Geometry check sheet. Reference: the model listing, model coordinates, mm. Face numbers are marked on the shaded views. A direction names the side the tool comes from. Give positions to 0.01 mm unless a question says otherwise; leave off trailing zeros. Loops run counter-clockwise (first coordinate to the right, second up) from the corner with the lowest first, then second, coordinate; pieces in that order, holes last. Notation, with made-up numbers: (76.25, 31.5) -> (81.25, 31.5) arc R20 cw to (81.25, 58.5) -> close; hole circle Ø1 at (-31.5, -27). An arc over 180 degrees is marked (long way). Write item = value, one per line. Start each with the question number.
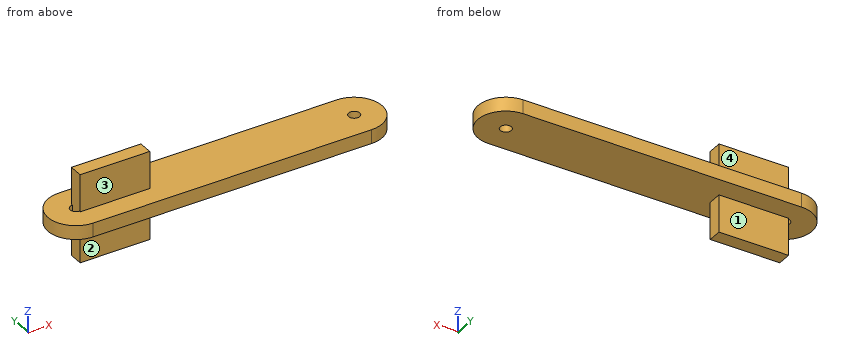
```python
from build123d import *

# Parameters (mm, degrees)
BOSS_EXTRUDE1_DEPTH      = 2.5
BOSS_EXTRUDE1_DEPTH_BACK = 2.5
SKETCH1_R                = 2
BOSS_EXTRUDE2_START      = -50
SKETCH2_W                = 31.75
SKETCH2_H                = 5
BOSS_EXTRUDE2_DEPTH      = 25


with BuildPart() as part:
    # Sketch1 → Boss-Extrude1 (new, two sides: drawn at the far end of the back side and taken through both)
    with BuildSketch(Plane.XY.offset(-BOSS_EXTRUDE1_DEPTH_BACK)):
        with BuildLine():
            Line((-50, 10), (50, 10))
            ThreePointArc((50, 10), (60, 0), (50, -10))
            Line((50, -10), (-50, -10))
            ThreePointArc((-50, -10), (-60, 0), (-50, 10))
        make_face()
        with Locations((-50, 0)):
            Circle(SKETCH1_R, mode=Mode.SUBTRACT)
        with Locations((50, 0)):
            Circle(SKETCH1_R, mode=Mode.SUBTRACT)
    extrude(amount=BOSS_EXTRUDE1_DEPTH + BOSS_EXTRUDE1_DEPTH_BACK)

    # Sketch2 → Boss-Extrude2 (add)
    with BuildSketch(Plane(origin=(0, 0, 0), x_dir=(0, 0, -1), z_dir=(1, 0, 0)).offset(BOSS_EXTRUDE2_START)):
        Rectangle(SKETCH2_W, SKETCH2_H)
    extrude(amount=BOSS_EXTRUDE2_DEPTH)


solid = part.part
```
1) Section check D-D (x = 40). Enter the section's corners in (y, z), plus the area to 3 significant figures.
2) Section check C-C (z = 7). Enter the section's corners in (x, y), plus the area to 3 significant figures.
3) Section check A-A (y = 0). Enter the section's corners in (x, z) (3 decimals).
4) Thickness scan on line 1 (Y direction, x = 50, z = -1); line 2 (Z direction, x = 0, y = -5.75); line 3 (X direction, y = 1, z = -12). Record the ranges inside material, lowest first.
5) Tool access check on the marked faces 1, 2, 3 and 4. Record the directions out of +Z, -Z, +X, -X, +Y, -Y that give a thin tool (end or side, any length) a straight path to the whole face; none if there is none.
6) Section check B-B (x = -32). Enter the section's corners in (y, z) (3 decimals), plus the area to 3 significant figures.
7) Depth check by flat-ended pin: pin 1 Ø1.5 at (y, z) = (1, -7) entering from +X; pin 2 Ø3 at (y, z) = (5.5, -7.5) entering from +X; pin 3 Ø1.5 at (x, z) = (-27.5, -7) entering from +Y; pin 4 Ø1.5 at (y, z) = (-1, 4) entering from -X. Enter the tip coordinate at first touch or a pass-through.
Check result:
q1.outline = (-10, -2.5) -> (10, -2.5) -> (10, 2.5) -> (-10, 2.5) -> close
q1.area = 100 mm2
q2.outline = (-50, -2.5) -> (-25, -2.5) -> (-25, 2.5) -> (-50, 2.5) -> close
q2.area = 125 mm2
q3.outline = (-60, -2.5) -> (-52, -2.5) -> (-52, 2.5) -> (-60, 2.5) -> close; (-50, -15.875) -> (-25, -15.875) -> (-25, -2.5) -> (48, -2.5) -> (48, 2.5) -> (-25, 2.5) -> (-25, 15.875) -> (-50, 15.875) -> close; (52, -2.5) -> (60, -2.5) -> (60, 2.5) -> (52, 2.5) -> close
q4.line_1 = -10 to -2, 2 to 10
q4.line_2 = -2.5 to 2.5
q4.line_3 = -50 to -25
q5.face_1 = -Z, +X, -X, +Y
q5.face_2 = -Z, +X, -X, -Y
q5.face_3 = +Z, +X, -X, -Y
q5.face_4 = +Z, +X, -X, +Y
q6.outline = (-10, -2.5) -> (-2.5, -2.5) -> (-2.5, -15.875) -> (2.5, -15.875) -> (2.5, -2.5) -> (10, -2.5) -> (10, 2.5) -> (2.5, 2.5) -> (2.5, 15.875) -> (-2.5, 15.875) -> (-2.5, 2.5) -> (-10, 2.5) -> close
q6.area = 234 mm2
q7.pin_1 = -25
q7.pin_2 = through
q7.pin_3 = 2.5
q7.pin_4 = -50
